Could you check a few things on this model? Use its own coordinates, in mm. Face numbers are marked on the shaded views. Coordinates: 2 decimals unless noted, no trailing zeros. Write each loop counter-clockwise with the first axis right and the second up, starting at its lowest first coordinate (ties: lowest second). Pieces come first, ordered by that corner, then holes. Notation, with made-up numbers: (61.25, 89) - (110.25, 89) arc R20 cw to (110.25, 103) - close; hole circle Ø5 at (76.25, -18.75). An arc over 180 degrees is marked (long way). Write item = value, one per line. Start each with the question number.
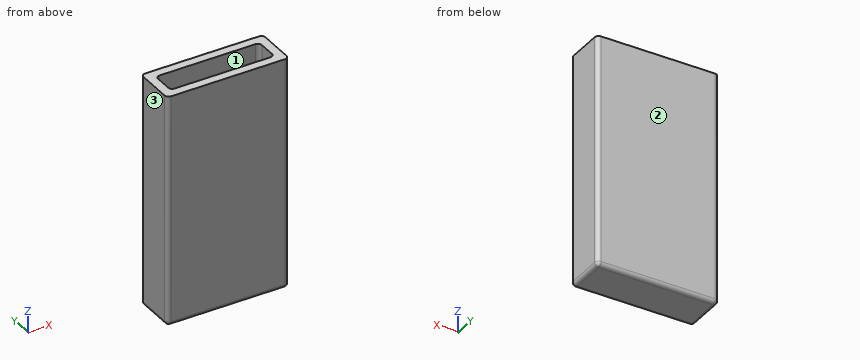
```python
from build123d import *

# Parameters (mm, degrees)
F0_W     = 31.75
F0_H     = 11.1125
F1_DEPTH = 60.325
F2_W     = 27.0256
F2_H     = 6.3881
F3_DEPTH = 57.9628
F4_R     = 1.016


with BuildPart() as f1:
    # F0 (on Top) → F1 (new body)
    with BuildSketch(Plane.XY):
        Rectangle(F0_W, F0_H)
    extrude(amount=F1_DEPTH)

    # F2 (on face) → F3 (cut)
    with BuildSketch(Plane.XY.offset(60.325)):
        Rectangle(F2_W, F2_H)
    extrude(amount=-F3_DEPTH, mode=Mode.SUBTRACT)

    # F4
    f4_edges = [f1.edges().sort_by_distance(p)[0] for p in [
        (-15.875, -5.55625, 30.1625),
        (15.875, -5.55625, 30.1625),
        (15.875, 5.55625, 30.1625),
        (-15.875, 5.55625, 30.1625),
        (13.5128, 3.19405, 31.3436),
        (-13.5128, 3.19405, 31.3436),
        (-13.5128, -3.19405, 31.3436),
        (13.5128, -3.19405, 31.3436),
        (0, -5.55625, 0),
        (15.875, 0, 0),
        (0, 5.55625, 0),
        (-15.875, 0, 0),
    ]]
    fillet(f4_edges, radius=F4_R)


solid = f1.part
```
1) Thinking about a two-plate mould opening in Y: for the marked faces 1, 2 and 3, which applies, +Y half, -Y half, draft (parallel to the pull), parting line (faces both ways), or undercut?
2) Suppose I cut it at A-A on z = 26.5. Please give me the cut outline in (x, y) (3 decimals), plus the area to 3 significant figures.
3) For P1, Ø3, axis at x = -4.5, y = -0.5, coming from the +Z side, with a flat end and sliding along its axis, tell me the tip position at first contact or that it passes through.
4) If I drill on probe 1 along Y at (x, z) = (-1, 22.5); probe 2 along X at (y, z) = (-2, 7) (3 decimals); probe 3 along Z at (x, y) = (2.5, 1.25), over which ranges is the centre line in solid material (lowest first)? Write a range as [from, to].
5) Suppose I cut it at C-C on x = 10. Please give me the cut outline in (y, z) (3 decimals), plus the area to 3 significant figures.
6) Suppose I cut it at B-B on y = -1.5. Please give me the cut outline in (x, z) (3 decimals), plus the area to 3 significant figures.
Reply:
q1.face_1 = undercut
q1.face_2 = +Y half
q1.face_3 = draft
q2.outline = (-15.875, -4.54) arc R1.016 ccw to (-14.859, -5.556) - (14.859, -5.556) arc R1.016 ccw to (15.875, -4.54) - (15.875, 4.54) arc R1.016 ccw to (14.859, 5.556) - (-14.859, 5.556) arc R1.016 ccw to (-15.875, 4.54) - close; hole (-13.513, -2.178) arc R1.016 ccw to (-12.497, -3.194) - (12.497, -3.194) arc R1.016 ccw to (13.513, -2.178) - (13.513, 2.178) arc R1.016 ccw to (12.497, 3.194) - (-12.497, 3.194) arc R1.016 ccw to (-13.513, 2.178) - close
q2.area = 180 mm^2
q3.P1 = 2.36
q4.probe_1 = [-5.56, -3.19], [3.19, 5.56]
q4.probe_2 = [-15.875, -13.513], [13.513, 15.875]
q4.probe_3 = [0, 2.36]
q5.outline = (-5.556, 1.016) arc R1.016 ccw to (-4.54, 0) - (4.54, 0) arc R1.016 ccw to (5.556, 1.016) - (5.556, 60.325) - (3.194, 60.325) - (3.194, 2.362) - (-3.194, 2.362) - (-3.194, 60.325) - (-5.556, 60.325) - close
q5.area = 300 mm^2
q6.outline = (-15.875, 1.016) arc R1.016 ccw to (-14.859, 0) - (14.859, 0) arc R1.016 ccw to (15.875, 1.016) - (15.875, 60.325) - (13.513, 60.325) - (13.513, 2.362) - (-13.513, 2.362) - (-13.513, 60.325) - (-15.875, 60.325) - close
q6.area = 348 mm^2
